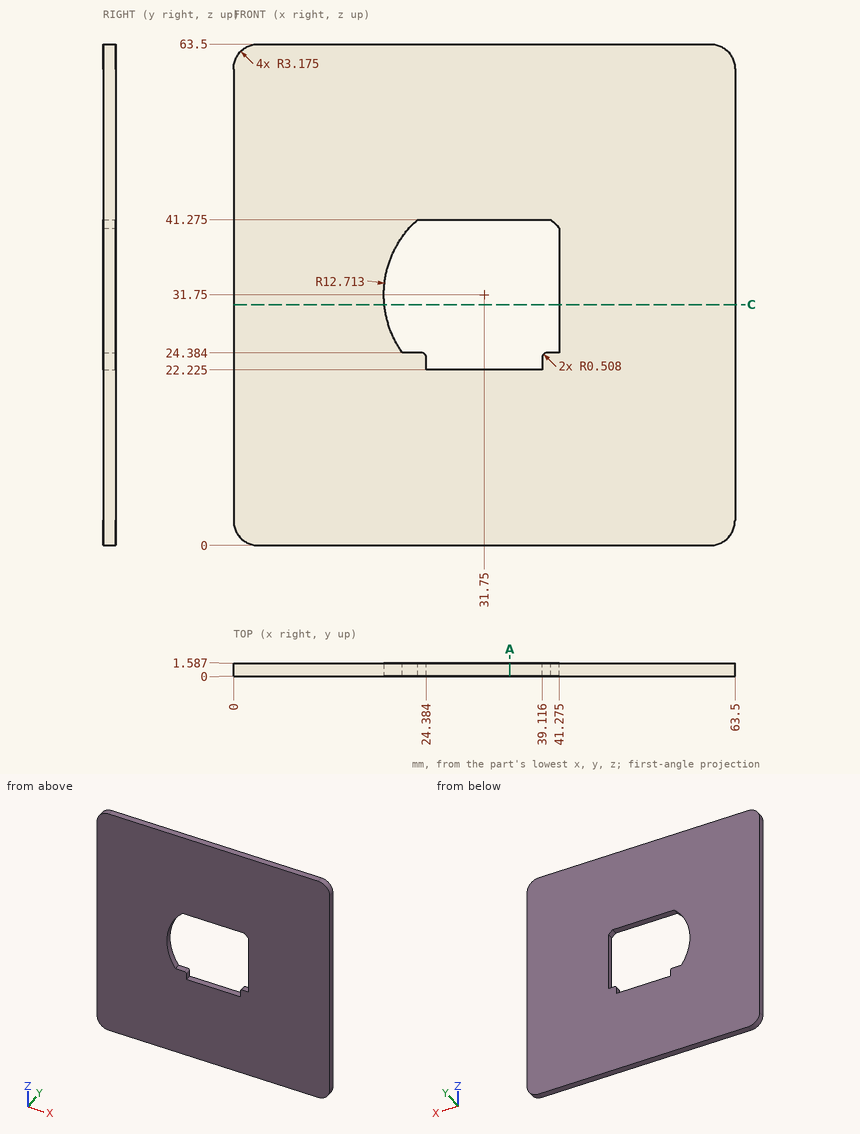
Part print with two shaded views. Sizes in mm from the minimum x, y, z corner. Coordinates: 2 decimals unless noted, no trailing zeros. Loops run counter-clockwise (first coordinate to the right, second up) from the corner with the lowest first, then second, coordinate; pieces in that order, holes last. Notation, with made-up numbers: (4, 25) - (18, 25) arc R21 cw to (18, 40) - close; hole circle Ø4 at (77.25, 71). An arc over 180 degrees is marked (long way). Write each question's results on one line, items separated by ' | '. Start each with the question number.
Q1. Probe line 1 along X through (y, z) = (0.1, 23) (1 decimal); line 2 along Z through (x, y) = (27.5, 0.25) (1 decimal); line 3 along X through (y, z) = (0.35, 40) (1 decimal). List the from-to ranges inside material, lowest first.
Q2. Slice it at C-C on z = 30.5. Give the cut face in (x, y) (1 decimal).
Q3. Slice it at A-A on x = 35. Give the cut face in (y, z) (1 decimal).
Answer:
1) line 1: x = 0 to 24.4, 39.1 to 63.5 | line 2: z = 0 to 22.2, 41.3 to 63.5 | line 3: x = 0 to 22.1, 41.3 to 63.5
2) outline: (0, 0) - (19.1, 0) - (19.1, 1.6) - (0, 1.6) - close; (41.3, 0) - (63.5, 0) - (63.5, 1.6) - (41.3, 1.6) - close
3) outline: (0, 0) - (1.6, 0) - (1.6, 22.2) - (0, 22.2) - close; (0, 41.3) - (1.6, 41.3) - (1.6, 63.5) - (0, 63.5) - close
